Geometry: see drawing. Coordinates: mm, zero at the bounding-box minimum. Round coordinates to 2 decimals unless told otherwise and drop trailing zeros. Order: outer loops, then holes, each group sorted by start corner. A loop starts at its lowest first (then second) coordinate and runs counter-clockwise, first axis right, second up. Notation, with made-up numbers: (-25.75, -13) -> (-20.75, -13) arc R16 ccw to (-20.75, 8) -> close; hole circle Ø4 at (-4.5, -12). An arc over 180 degrees is marked (long way). Write item = value, one per line. Start each with the question number.
(1) Contact query for flat-ended pins moving along their axis: pin 1 Ø3 at (x, z) = (0.5, 13) entering from -Y; pin 2 Ø3 at (x, z) = (3.5, 42) entering from +Y. Output: stop coordinate, or through.
(2) Cut plane A-A on x = 2.5. Return the cut outline in (y, z).
(3) Cut plane C-C on z = 28.5. Return the cut outline in (x, y), then the cut area to 3 significant figures.
(4) Ray query, line 1 (Z direction, x = 4.5, y = 2.35); line 2 (X direction, y = 2.4, z = 15). Return the intervals inside material, ascending.
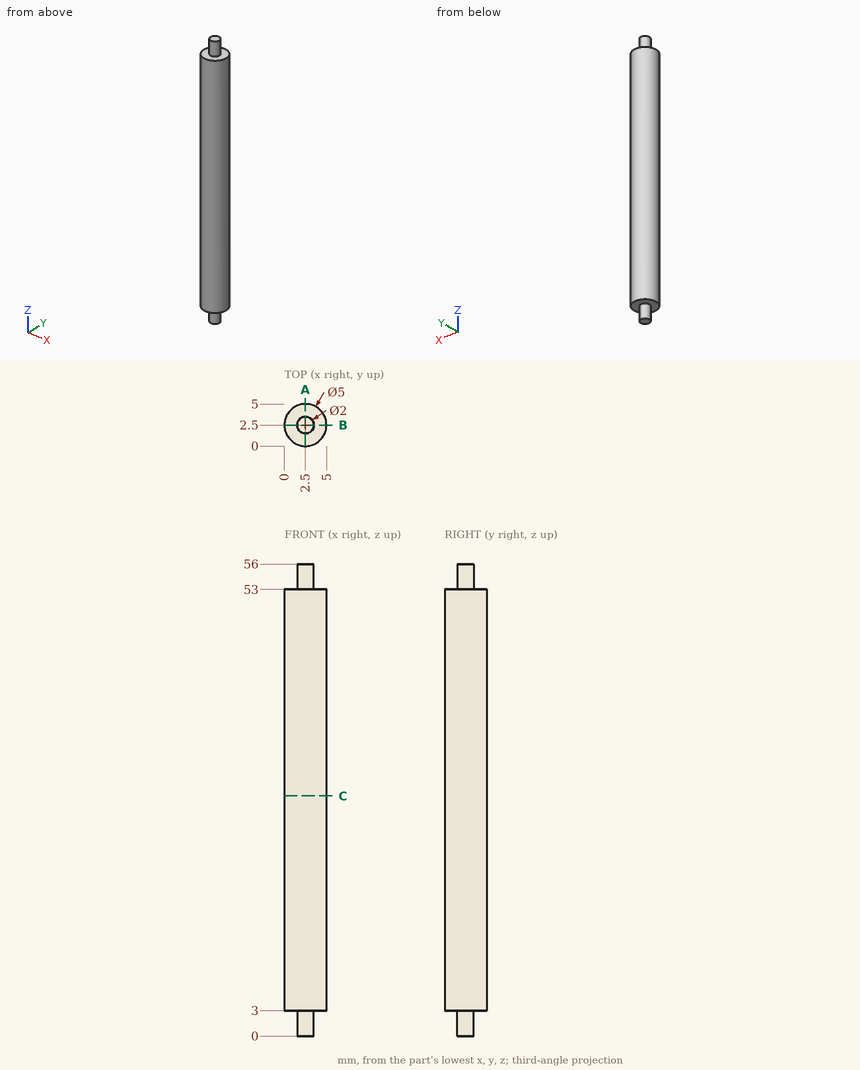
Evaluation:
q1.pin_1 = 0.05
q1.pin_2 = 5
q2.outline = (0, 3) -> (1.5, 3) -> (1.5, 0) -> (3.5, 0) -> (3.5, 3) -> (5, 3) -> (5, 53) -> (3.5, 53) -> (3.5, 56) -> (1.5, 56) -> (1.5, 53) -> (0, 53) -> close
q3.outline = circle Ø5 at (2.5, 2.5)
q3.area = 19.6 mm^2
q4.line_1 = 3 to 53
q4.line_2 = 0 to 5
